Design review of the part built by this model. Coordinates are the model's own, in mm. A direction names the side the tool comes from. Round coordinates to 2 decimals unless told otherwise and drop trailing zeros. Order: outer loops, then holes, each group sorted by start corner. A loop starts at its lowest first (then second) coordinate and runs counter-clockwise, first axis right, second up. Notation, with made-up numbers: (71, 20) - (78, 20) arc R9 cw to (78, 30) - close; hole circle Ø5 at (58, -26). An arc over 180 degrees is marked (long way). Use CSV: the item, a comma, the result in double quotes.
from build123d import *

# Parameters (mm, degrees)
SKETCH1_R           = 37
BOSS_EXTRUDE1_DEPTH = 150
SKETCH2_W           = 23
SKETCH2_H           = 23
CUT_EXTRUDE1_DEPTH  = 150
SKETCH3_W           = 43
SKETCH3_H           = 43
CUT_EXTRUDE2_DEPTH  = 36
CHAMFER1_SIZE       = 5
SKETCH5_R           = 32.5
CUT_EXTRUDE3_DEPTH  = 15
SKETCH11_W          = 44.607289856
SKETCH11_H          = 47.277792796
CUT_EXTRUDE7_DEPTH  = 104
SKETCH12_W          = 26
SKETCH12_H          = 20
BOSS_EXTRUDE2_DEPTH = 10
SKETCH13_W          = 20
SKETCH13_H          = 31
CUT_EXTRUDE8_DEPTH  = 11
SKETCH14_W          = 20
SKETCH14_H          = 10
BOSS_EXTRUDE3_DEPTH = 10
SKETCH15_W          = 20
SKETCH15_H          = 10
BOSS_EXTRUDE4_DEPTH = 10


with BuildPart() as part:
    # Sketch1 → Boss-Extrude1 (new body)
    with BuildSketch(Plane(origin=(0, 0, 0), x_dir=(1, 0, 0), z_dir=(0, 1, 0))):
        with Locations(Location((0, 0, 0), (0, 0, 270))):
            Circle(SKETCH1_R)
    extrude(amount=BOSS_EXTRUDE1_DEPTH)

    # Sketch2 → Cut-Extrude1 (cut)
    with BuildSketch(Plane(origin=(0, 150, 0), x_dir=(1, 0, 0), z_dir=(0, 1, 0))):
        Rectangle(SKETCH2_W, SKETCH2_H)
    extrude(amount=-CUT_EXTRUDE1_DEPTH, mode=Mode.SUBTRACT)

    # Sketch3 → Cut-Extrude2 (cut)
    with BuildSketch(Plane.XZ):
        Rectangle(SKETCH3_W, SKETCH3_H)
    extrude(amount=-CUT_EXTRUDE2_DEPTH, mode=Mode.SUBTRACT)

    # Chamfer1
    chamfer1_edges = [part.edges().sort_by_distance(p)[0] for p in [
        (21.5, 18, 21.5),
        (21.5, 18, -21.5),
        (-21.5, 18, -21.5),
        (-21.5, 18, 21.5),
    ]]
    chamfer(chamfer1_edges, length=CHAMFER1_SIZE)

    # Sketch5 → Cut-Extrude3 (cut)
    with BuildSketch(Plane(origin=(0, 150, 0), x_dir=(1, 0, 0), z_dir=(0, 1, 0))):
        with Locations(Location((0, 0, 0), (0, 0, 270))):
            Circle(SKETCH5_R)
    extrude(amount=-CUT_EXTRUDE3_DEPTH, mode=Mode.SUBTRACT)

    # Sketch11 → Cut-Extrude7 (cut)
    with BuildSketch(Plane(origin=(0, 135, 0), x_dir=(1, 0, 0), z_dir=(0, 1, 0))):
        Rectangle(SKETCH11_W, SKETCH11_H)
    extrude(amount=-CUT_EXTRUDE7_DEPTH, mode=Mode.SUBTRACT)

    # Sketch12 → Boss-Extrude2 (add)
    with BuildSketch(Plane.XZ):
        with Locations((-34.5, 0)):
            Rectangle(SKETCH12_W, SKETCH12_H)
        with Locations((34.5, 0)):
            Rectangle(SKETCH12_W, SKETCH12_H)
    extrude(amount=-BOSS_EXTRUDE2_DEPTH)

    # Sketch13 → Cut-Extrude8 (cut)
    with BuildSketch(Plane.XZ):
        with Locations((0, 37)):
            Rectangle(SKETCH13_W, SKETCH13_H)
    extrude(amount=-CUT_EXTRUDE8_DEPTH, mode=Mode.SUBTRACT)

    # Sketch14 → Boss-Extrude3 (add)
    with BuildSketch(Plane(origin=(47.5, 0, 0), x_dir=(0, 0, -1), z_dir=(1, 0, 0))):
        with Locations((0, 5)):
            Rectangle(SKETCH14_W, SKETCH14_H)
    extrude(amount=BOSS_EXTRUDE3_DEPTH)

    # Sketch15 → Boss-Extrude4 (add)
    with BuildSketch(Plane.ZY.offset(47.5)):
        with Locations((0, 5)):
            Rectangle(SKETCH15_W, SKETCH15_H)
    extrude(amount=BOSS_EXTRUDE4_DEPTH)


solid = part.part
1) We need section B-B (y = 26.5). Give the boundary of the cut face in (x, z).
Data:
outline,"circle Ø74 at (0, 0); hole (-21.5, -16.5) - (-16.5, -21.5) - (16.5, -21.5) - (21.5, -16.5) - (21.5, 16.5) - (16.5, 21.5) - (-16.5, 21.5) - (-21.5, 16.5) - close"
2) We need section A-A (z = 0). Give the boundary of the cut face in (x, y), then the cut area to 3 significant figures.
Data:
outline,"(-57.5, 0) - (-21.5, 0) - (-21.5, 31) - (-22.3, 31) - (-22.3, 135) - (-32.5, 135) - (-32.5, 150) - (-37, 150) - (-37, 10) - (-57.5, 10) - close; (21.5, 0) - (57.5, 0) - (57.5, 10) - (37, 10) - (37, 150) - (32.5, 150) - (32.5, 135) - (22.3, 135) - (22.3, 31) - (21.5, 31) - close"
area,"4,560 mm2"
3) The part is to be moulded in two halves that separate along X. For faces 1 (the face through (-14.17, 73.95, 34.18)), 2 (the face through (-22, 31, 2)), 3 (the face through (46, 5, -10)), say which applies: +X half, -X half, draft (parallel to the pull), parting line (faces both ways), or undercut.
Data:
face 1,"parting line"
face 2,"undercut"
face 3,"draft"
4) We need section D-D (x = -28). Give the boundary of the cut face in (y, z).
Data:
outline,"(0, -24.19) - (150, -24.19) - (150, -16.5) - (135, -16.5) - (135, 16.5) - (150, 16.5) - (150, 24.19) - (0, 24.19) - close"
5) We need section C-C (x = 0). Give the boundary of the cut face in (y, z), then the cut area to 3 significant figures.
Data:
outline,"(0, -37) - (150, -37) - (150, -32.5) - (135, -32.5) - (135, -23.64) - (31, -23.64) - (31, -21.5) - (0, -21.5) - close; (11, 21.5) - (31, 21.5) - (31, 23.64) - (135, 23.64) - (135, 32.5) - (150, 32.5) - (150, 37) - (11, 37) - close"
area,"3,700 mm2"
6) For faces 4 (the face through (-19, 15, -19)), 5 (the face through (-46, 5, -10)), 6 (the face through (-22.304, 84, 0)), list the 3-axis set-ups (+Z, -Z, +X, -X, +Y, -Y) from which the entire face can be reached by the end or side of a thin tool; tool diameter is ignored.
Data:
face 4,"+Y, -Y"
face 5,"-Z, -X, +Y, -Y"
face 6,"+Y"
7) Insertion check: pin 1 Ø12 at (y, z) = (60, -19.5) entering from -X; pin 2 Ø8 at (y, z) = (97, 11.5) entering from +X; pin 3 Ø4.5 at (x, z) = (-1, 27.5) entering from -Y. Each pin has a flat end and moves straight along its axis. Give the tip position at first contact, or say it passes through.
Data:
pin 1,"stops at x = -34.45"
pin 2,"stops at x = 36.23"
pin 3,"stops at y = 11"
8) To check wall thickness, follow L1, parallel to X at y = 138, z = 0; L2, parallel to X at y = 141, z = 17.5. State the ranges of each line that lie inside material, in increasing order. Write a range as from..to.
Data:
L1,"x = -37..-32.5, 32.5..37"
L2,"x = -32.6..-27.39, 27.39..32.6"
